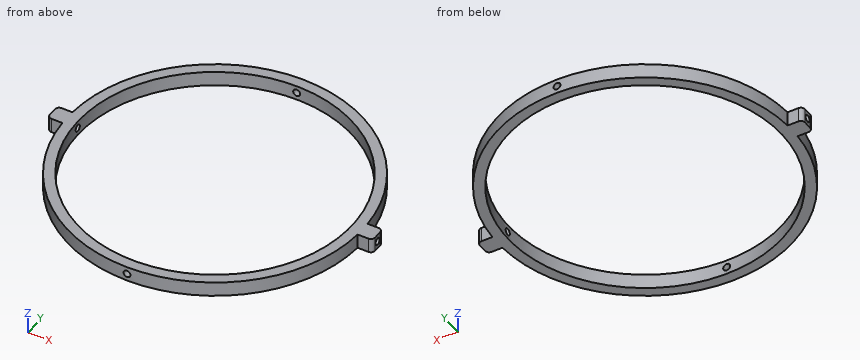
```python
from build123d import *

# Parameters (mm, degrees)
SKETCH071_R          = 70
SKETCH071_R_2        = 65
SKETCH071_W          = 12
SKETCH071_H          = 8
PAD004_DEPTH         = 3.5
PAD005_DEPTH         = 3.5
SKETCH073_R          = 1.65
POCKET003_DEPTH      = 70.001
POCKET003_DEPTH_BACK = 70.001
SKETCH084_R          = 1.65
POCKET010_DEPTH      = 77.001
POCKET010_DEPTH_BACK = 77.001
FILLET002_R          = 2


with BuildPart() as part:
    # Sketch071 → Pad004 (new body, symmetric)
    with BuildSketch(Plane.XY):
        Circle(SKETCH071_R)
        Circle(SKETCH071_R_2, mode=Mode.SUBTRACT)
        with Locations((71, 0)):
            Rectangle(SKETCH071_W, SKETCH071_H)
        with Locations((-71, 0)):
            Rectangle(SKETCH071_W, SKETCH071_H)
    extrude(amount=PAD004_DEPTH, both=True)

    # Sketch071 → Pad005 (join, symmetric)
    with BuildSketch(Plane.XY):
        Circle(SKETCH071_R)
        Circle(SKETCH071_R_2, mode=Mode.SUBTRACT)
        with Locations((71, 0)):
            Rectangle(SKETCH071_W, SKETCH071_H)
        with Locations((-71, 0)):
            Rectangle(SKETCH071_W, SKETCH071_H)
    extrude(amount=PAD005_DEPTH, both=True)

    # Sketch073 → Pocket003 (cut, two sides)
    with BuildSketch(Plane.XZ) as pocket003_sk:
        Circle(SKETCH073_R)
    extrude(amount=-POCKET003_DEPTH, mode=Mode.SUBTRACT)
    extrude(pocket003_sk.sketch, amount=POCKET003_DEPTH_BACK, mode=Mode.SUBTRACT)

    # Sketch084 → Pocket010 (cut, two sides)
    with BuildSketch(Plane.YZ) as pocket010_sk:
        Circle(SKETCH084_R)
    extrude(amount=-POCKET010_DEPTH, mode=Mode.SUBTRACT)
    extrude(pocket010_sk.sketch, amount=POCKET010_DEPTH_BACK, mode=Mode.SUBTRACT)

    # Fillet002
    fillet002_edges = [part.edges().sort_by_distance(p)[0] for p in [
        (77, -4, 0),
        (77, 4, 0),
        (-77, -4, 0),
        (-77, 4, 0),
    ]]
    fillet(fillet002_edges, radius=FILLET002_R)


solid = part.part
```
Geometry: final body of the model. Coordinates: model frame, mm. Round coordinates to 2 decimals unless told otherwise and drop trailing zeros. Write each loop counter-clockwise with the first axis right and the second up, starting at its lowest first coordinate (ties: lowest second). Pieces come first, ordered by that corner, then holes. Notation, with made-up numbers: (11, -33.75) -> (40, -33.75) arc R17 ccw to (40, -24.75) -> close; hole circle Ø9 at (35.25, -26). An arc over 180 degrees is marked (long way). Return JSON: item names as keys, results as strings.
Q1. Section A-A on x = -33.5. Return the cut outline in (y, z), and give its area (3 significant figures).
From the geometry:
{"outline": "(-61.46, -3.5) -> (-55.7, -3.5) -> (-55.7, 3.5) -> (-61.46, 3.5) -> close; (55.7, -3.5) -> (61.46, -3.5) -> (61.46, 3.5) -> (55.7, 3.5) -> close", "area": "80.7 mm2"}
Q2. Ray query, line 1 (Z direction, x = 0, y = 66.2); line 2 (Y direction, x = 0, z = 1.75); line 3 (Y direction, x = -57.5, z = 2.25). Return the intervals inside material, ascending.
From the geometry:
{"line 1": "-3.5 to -1.65, 1.65 to 3.5", "line 2": "-70 to -65, 65 to 70", "line 3": "-39.92 to -30.31, 30.31 to 39.92"}
Q3. Section B-B on z = 0. Return the cut outline in (x, y), and give its area (3 significant figures).
From the geometry:
{"outline": "(-77, -2) arc R2 ccw to (-75, -4) -> (-69.89, -4) arc R70 ccw to (-1.65, -69.98) -> (-1.65, -64.98) arc R65 cw to (-64.98, -1.65) -> (-77, -1.65) -> close; (-77, 1.65) -> (-64.98, 1.65) arc R65 cw to (-1.65, 64.98) -> (-1.65, 69.98) arc R70 ccw to (-69.89, 4) -> (-75, 4) arc R2 ccw to (-77, 2) -> close; (1.65, -69.98) arc R70 ccw to (69.89, -4) -> (75, -4) arc R2 ccw to (77, -2) -> (77, -1.65) -> (64.98, -1.65) arc R65 cw to (1.65, -64.98) -> close; (1.65, 64.98) arc R65 cw to (64.98, 1.65) -> (77, 1.65) -> (77, 2) arc R2 ccw to (75, 4) -> (69.89, 4) arc R70 ccw to (1.65, 69.98) -> close", "area": "2,120 mm2"}
Q4. First-contact query: pin 1 Ø1.5 at (x, z) = (-71.5, 1) entering from +Y. Flat tip, straight axial feed; report the tip coordinate or a pass-through.
From the geometry:
{"pin 1": "y = 4"}
Q5. Section C-C on y = -50. Return the cut outline in (x, z).
From the geometry:
{"outline": "(-48.99, -3.5) -> (-41.53, -3.5) -> (-41.53, 3.5) -> (-48.99, 3.5) -> close; (41.53, -3.5) -> (48.99, -3.5) -> (48.99, 3.5) -> (41.53, 3.5) -> close"}
